Part print with two shaded views. Sizes in mm from the minimum x, y, z corner. A direction names the side the tool comes from. Give positions to 0.01 mm unless a question says otherwise; leave off trailing zeros. Write each loop counter-clockwise with the first axis right and the second up, starting at its lowest first coordinate (ties: lowest second). Pieces come first, ordered by that corner, then holes. Notation, with made-up numbers: (-17.75, 80) - (1.25, 80) arc R26 cw to (1.25, 114) - close; hole circle Ø3 at (61.5, 26.5). An arc over 180 degrees is marked (long way). Answer as a JSON object with one key per item and string values.
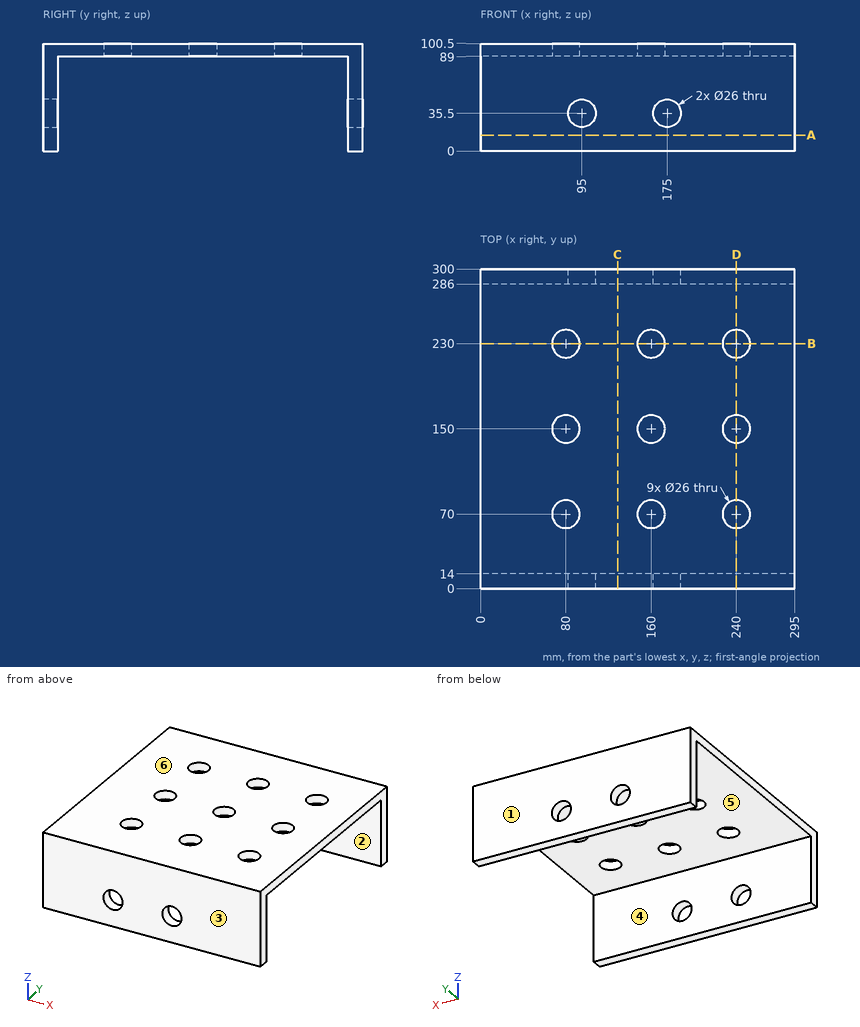
(1) Saw through at B-B, the plane y = 230. Give the cut face in (x, z), and give its area (3 significant figures).
Answer key:
{"outline": "(0, 89) - (67, 89) - (67, 100.5) - (0, 100.5) - close; (93, 89) - (147, 89) - (147, 100.5) - (93, 100.5) - close; (173, 89) - (227, 89) - (227, 100.5) - (173, 100.5) - close; (253, 89) - (295, 89) - (295, 100.5) - (253, 100.5) - close", "area": "2,500 mm²"}
(2) Pull direction Y, two halves, no side cores. Call the marked faces 3, 4, 5 and 6: pulls with the +Y half, pulls with the -Y half, needs draft (parallel to the pull), parting line crosses it, or undercut.
Answer key:
{"face 3": "pulls with the -Y half", "face 4": "undercut", "face 5": "undercut", "face 6": "needs draft"}
(3) Saw through at A-A, the plane z = 15. Give the cut face in (x, y).
Answer key:
{"outline": "(0, 0) - (295, 0) - (295, 14) - (0, 14) - close; (0, 286) - (295, 286) - (295, 300) - (0, 300) - close"}
(4) Saw through at D-D, the plane x = 240. Give the cut face in (y, z).
Answer key:
{"outline": "(0, 0) - (14, 0) - (14, 89) - (57, 89) - (57, 100.5) - (0, 100.5) - close; (83, 89) - (137, 89) - (137, 100.5) - (83, 100.5) - close; (163, 89) - (217, 89) - (217, 100.5) - (163, 100.5) - close; (243, 89) - (286, 89) - (286, 0) - (300, 0) - (300, 100.5) - (243, 100.5) - close"}
(5) Saw through at C-C, the plane x = 128.5. Give the cut face in (y, z).
Answer key:
{"outline": "(0, 0) - (14, 0) - (14, 89) - (286, 89) - (286, 0) - (300, 0) - (300, 100.5) - (0, 100.5) - close"}
(6) 3-axis set-ups, long thin cutter, end or side, ignore diameter. For the marked faces 1 and 2: which of +Z, -Z, +X, -X, +Y, -Y reach the whole face in a straight line?
Answer key:
{"face 1": "+Z, -Z, +X, -X, +Y", "face 2": "-Z, +X, -X"}
(7) Probe L1, parallel to Y at x = 80, z = 92; L2, parallel to X at y = 297.25, z = 35.5; L3, parallel to Y at x = 46.5, z = 47. List the from-to ranges inside material, lowest first. Write a range as [from, to].
Answer key:
{"L1": "y = [0, 57], [83, 137], [163, 217], [243, 300]", "L2": "x = [0, 82], [108, 162], [188, 295]", "L3": "y = [0, 14], [286, 300]"}
(8) Flat gauge pin, fed straight in: P1, Ø10, axis at x = 68.5, y = 197, coming from the -Z side. Where does the tip first touch, or does it go through?
Answer key:
{"P1": "stops at z = 89"}
